Part model, mm, in its own coordinate system. A direction names the side the tool comes from. Give positions to 0.01 mm unless a question says otherwise; leave off trailing zeros. Order: outer loops, then holes, each group sorted by start corner. A loop starts at its lowest first (then second) coordinate and runs counter-clockwise, first axis right, second up.
1. Slice it at C-C on z = 0. List the corners of the cut face in (x, y).
2. Drop flat-ended pins along their axis: pin 1 Ø2 at (x, y) = (-4.5, 2) entering from -Z; pin 2 Ø1.5 at (y, z) = (-0.5, -3) entering from -X; pin 3 Ø3 at (x, z) = (-5, 0) entering from +Y. Give the stop position or say it passes through.
3. Slice it at D-D on z = -3. List the corners of the cut face in (x, y), and give its area (3 significant figures).
4. Probe line 1 (Y direction, x = -7, z = -3); line 2 (X direction, y = -2.55, z = 0); line 3 (Z direction, x = 6.25, y = 3.5). List the from-to ranges inside material, lowest first.
5. Slice it at A-A on x = -4.75. List the corners of the cut face in (y, z).
6. Mould opens along Z. For faces 5 (the cylindrical face through (5.578, -3.43, 7.696)), 6 (the flat face through (-4, -2, -5)), 7 (the flat face through (-4, -3, 2)) say: +Z half, -Z half, draft (parallel to the pull), parting line (faces both ways), or undercut.
7. Slice it at B-B on y = -0.5. List the corners of the cut face in (x, z).
8. Which spindle directions (+Z, -Z, +X, -X, +Y, -Y) get a long thin tool onto all of the face, cutting with end or side? Do faces 1 (the flat face through (-4, 2, -5)), 2 (the flat face through (-4, 3, 2)), 3 (the flat face through (1, 0, 5)), 4 (the flat face through (0, 0, 4)). Say none if no direction does.
from build123d import *

# Parameters (mm, degrees)
BOSS_EXTRUDE1_DEPTH          = 5
SKETCH2_R                    = 5
SKETCH2_R_2                  = 1.4
BOSS_EXTRUDE2_DEPTH          = 1.5
BOSS_EXTRUDE3_REACH          = 13.576
SKETCH4_W                    = 10
SKETCH4_H                    = 1.5
SKETCH6_R                    = 5
SKETCH6_R_2                  = 1.4
BOSS_EXTRUDE4_DEPTH          = 1.5
BOSS_EXTRUDE5_REACH          = 13.576
SKETCH5_W                    = 10
SKETCH5_H                    = 1.5
SCHIZZO1_W                   = 10
SCHIZZO1_H                   = 6
ESTRUSIONE_ESTRUSIONE2_DEPTH = 11
TAGLIO_ESTRUSIONE1_DEPTH     = 11
ESTRUSIONE_ESTRUSIONE3_DEPTH = 5
SCHIZZO4_R                   = 6
TAGLIO_ESTRUSIONE2_DEPTH     = 3


with BuildPart() as part:
    # Sketch1 → Boss-Extrude1 (new, symmetric)
    with BuildSketch(Plane.XY):
        with BuildLine():
            Line((0, 3), (0, 1.5))
            ThreePointArc((0, 1.5), (1.5, 0), (0, -1.5))
            Line((0, -1.5), (0, -3))
            ThreePointArc((0, -3), (3, 0), (0, 3))
        make_face()
    extrude(amount=BOSS_EXTRUDE1_DEPTH, both=True)


with BuildPart() as body_2:
    # Sketch2 → Boss-Extrude2 (new body)
    with BuildSketch(Plane(origin=(0, 1.5, 0), x_dir=(1, 0, 0), z_dir=(0, 1, 0))):
        with Locations(Location((-5, 0, 0), (0, 0, 270))):
            Circle(SKETCH2_R)
        with Locations(Location((-5, 0, 0), (0, 0, 270))):
            Circle(SKETCH2_R_2, mode=Mode.SUBTRACT)
    extrude(amount=BOSS_EXTRUDE2_DEPTH)

    # Sketch4 → Boss-Extrude3 (add, up to next)
    with BuildSketch(Plane.ZY, mode=Mode.PRIVATE) as boss_extrude3_sk1:
        with Locations((0, 2.25)):
            Rectangle(SKETCH4_W, SKETCH4_H)
    boss_extrude3_tool1 = extrude(boss_extrude3_sk1.sketch, amount=BOSS_EXTRUDE3_REACH, mode=Mode.PRIVATE) - body_2.part

    add(part.part)  # Boss-Extrude3 merges part
    add(boss_extrude3_tool1.solids().sort_by_distance((0, 2.25, 0))[0])
    add(boss_extrude3_tool1.solids().sort_by_distance((0, 2.25, 0))[1])


with BuildPart() as body_2_2:
    # Sketch6 → Boss-Extrude4 (new body)
    with BuildSketch(Plane(origin=(0, -1.5, 0), x_dir=(1, 0, 0), z_dir=(0, 1, 0))):
        with Locations(Location((-5, 0, 0), (0, 0, 270))):
            Circle(SKETCH6_R)
        with Locations(Location((-5, 0, 0), (0, 0, 270))):
            Circle(SKETCH6_R_2, mode=Mode.SUBTRACT)
    extrude(amount=-BOSS_EXTRUDE4_DEPTH)

    # Sketch5 → Boss-Extrude5 (add, up to next)
    with BuildSketch(Plane.ZY, mode=Mode.PRIVATE) as boss_extrude5_sk1:
        with Locations((0, -2.25)):
            Rectangle(SKETCH5_W, SKETCH5_H)
    boss_extrude5_tool1 = extrude(boss_extrude5_sk1.sketch, amount=BOSS_EXTRUDE5_REACH, mode=Mode.PRIVATE) - body_2_2.part

    add(body_2.part)  # Boss-Extrude5 merges body 2
    add(boss_extrude5_tool1.solids().sort_by_distance((0, -2.25, 0))[0])
    add(boss_extrude5_tool1.solids().sort_by_distance((0, -2.25, 0))[1])

    # Schizzo1 → Estrusione-Estrusione2 (add)
    with BuildSketch(Plane.ZY):
        Rectangle(SCHIZZO1_W, SCHIZZO1_H)
    extrude(amount=-ESTRUSIONE_ESTRUSIONE2_DEPTH)

    # Schizzo2 → Taglio-Estrusione1 (cut)
    with BuildSketch(Plane.XZ.offset(3)):
        Polygon((3, -5), (7.130949903, 5), (11, 5), (13.561973645, 5), (13.561973645, -5), align=None)
    extrude(amount=-TAGLIO_ESTRUSIONE1_DEPTH, mode=Mode.SUBTRACT)

    # Schizzo3 → Estrusione-Estrusione3 (add)
    with BuildSketch(Plane(origin=(4.327071195, 0, -1.787491434), x_dir=(-0.3818008251213657, 0, -0.9242446266744776), z_dir=(0.9242446266744775, 0, -0.38180082512136565))):
        with BuildLine():
            Line((-7.84382569, 4), (7.15617431, 4))
            Line((7.15617431, 4), (7.15617431, -4))
            Line((7.15617431, -4), (-7.84382569, -4))
            ThreePointArc((-7.84382569, -4), (-9.258039253, -3.414213562), (-9.84382569, -2))
            Line((-9.84382569, -2), (-9.84382569, 2))
            ThreePointArc((-9.84382569, 2), (-9.258039253, 3.414213562), (-7.84382569, 4))
        make_face()
    extrude(amount=-ESTRUSIONE_ESTRUSIONE3_DEPTH)

    # Schizzo4 → Taglio-Estrusione2 (cut)
    with BuildSketch(Plane.XZ.offset(-1.5)):
        with Locations((-5, 0)):
            Circle(SCHIZZO4_R)
    extrude(amount=TAGLIO_ESTRUSIONE2_DEPTH, mode=Mode.SUBTRACT)


solid = body_2_2.part
Data:
1. outline: (-10, -3) - (-6.4, -3) - (-6.4, -1.5) - (-10, -1.5) - close; (-10, 1.5) - (-6.4, 1.5) - (-6.4, 3) - (-10, 3) - close; (-3.6, -3) - (-0.34, -3) - (-0.34, -4) - (5.07, -4) - (5.07, 4) - (-0.34, 4) - (-0.34, 3) - (-3.6, 3) - (-3.6, 1.5) - (1, 1.5) - (1, -1.5) - (-3.6, -1.5) - close
2. pin 1: stops at z = -5
2. pin 2: stops at x = -0.32
2. pin 3: stops at y = 3
3. outline: (-9, -3) - (-1.58, -3) - (-1.58, -4) - (3.83, -4) - (3.83, 4) - (-1.58, 4) - (-1.58, 3) - (-9, 3) - (-9, 1.5) - (0.2, 1.5) - (0.2, -1.5) - (-9, -1.5) - close
3. area: 60.2 mm2
4. line 1: y = -3 to -1.5, 1.5 to 3
4. line 2: x = -10 to -6.4, -3.6 to 5.07
4. line 3: z = 2.87 to 7.34
5. outline: (-3, -5) - (-1.5, -5) - (-1.5, -1.38) - (-3, -1.38) - close; (-3, 1.38) - (-1.5, 1.38) - (-1.5, 5) - (-3, 5) - close; (1.5, -5) - (3, -5) - (3, -1.38) - (1.5, -1.38) - close; (1.5, 1.38) - (3, 1.38) - (3, 5) - (1.5, 5) - close
6. face 5: +Z half
6. face 6: undercut
6. face 7: draft
7. outline: (-3.03, -6.49) - (1.59, -8.4) - (8.09, 7.31) - (3.46, 9.22) - (1.72, 5) - (0, 5) - (0, 3.32) arc R6 cw to (-2.62, -5.51) - close
8. face 1: -X, +Y, -Y
8. face 2: +Z, -X, +Y
8. face 3: +Z, -X, +Y, -Y
8. face 4: +Z, -X
